Autodesk Inventor part; units mm, degrees
ref_plane "Work Plane2" through (32.2, 0, -89.46) normal (-1, 0, 0) x (0, 0, 1)
ref_plane "YZ Plane" through (0, 0, 0) normal (1, 0, 0) x (0, 1, 0)
ref_plane "XZ Plane" through (0, 0, 0) normal (0, 1, 0) x (-1, 0, 0)
sketch "Sketch1" plane through (0, 0, 0) normal (0, 1, 0) x (-1, 0, 0)
  line L0 (0, 0) -> (-11.7, 0)
  line L1 (-11.7, 0) -> (-11.7, -89.46)
  line L2 (-11.7, -89.46) -> (0, -89.46)
  line L3 (0, -89.46) -> (0, 0)
  line L4 (-26.35, 0) -> (-38.05, 0)
  line L5 (-38.05, 0) -> (-38.05, -89.46)
  line L6 (-38.05, -89.46) -> (-26.35, -89.46)
  line L7 (-26.35, -89.46) -> (-26.35, 0)
  line L8 (-52.7, 0) -> (-64.4, 0)
  line L9 (-64.4, 0) -> (-64.4, -89.46)
  line L10 (-64.4, -89.46) -> (-52.7, -89.46)
  line L11 (-52.7, -89.46) -> (-52.7, 0)
  dimension "d0" = 11.7
  dimension "d1" = 11.7
  dimension "d2" = 11.7
  dimension "d3" = 14.65
  dimension "d4" = 14.65
  dimension "d5" = 89.46
  dimension "d47" = 64.4
extrude "Extrusion1" add sketch "Sketch1" along normal blind 9
sketch "Sketch2" plane through (0, 9, 0) normal (0, 1, 0) x (1, 0, 0)
  line L0 (38.05, 89.46) -> (26.35, 89.46) construction
  line L1 (32.2, 89.46) -> (32.2, 0) construction
  line L2 (26.35, 0) -> (38.05, 0) construction
  line L3 (11.7, 89.46) -> (0, 89.46) construction
  line L4 (5.85, 89.46) -> (5.85, 0) construction
  line L5 (0, 0) -> (11.7, 0) construction
  circle A0 centre (5.85, 84.96) radius 1.5
  circle A1 centre (58.55, 84.96) radius 1.5
  dimension "d8" = 3
  dimension "d9" = 4.5
extrude "Extrusion2" cut sketch "Sketch2" against normal blind 8
sketch "Sketch3" plane through (11.7, 0, -89.46) normal (0, 0, -1) x (-1, 0, 0)
  line L0 (-14.65, 9) -> (-26.35, 9) construction
  line L1 (-20.5, 9) -> (-20.5, 0) construction
  line L2 (-14.65, 0) -> (-26.35, 0) construction
  line L3 (0, 0) -> (11.7, 0)
  line L4 (9.6, 0) -> (9.6, 6.9)
  line L5 (9.6, 6.9) -> (2.1, 6.9)
  line L6 (2.1, 6.9) -> (2.1, 0)
  line L7 (2.1, 0) -> (9.6, 0) construction
  line L8 (0, 0) -> (0, 9) construction
  line L9 (11.7, 0) -> (11.7, 9) construction
  line L10 (-41, 0) -> (-52.7, 0)
  line L11 (-50.6, 0) -> (-50.6, 6.9)
  line L12 (-50.6, 6.9) -> (-43.1, 6.9)
  line L13 (-43.1, 6.9) -> (-43.1, 0)
  dimension "d15" = 7.5
  dimension "d16" = 2.1
  dimension "d17" = 2.1
  dimension "d18" = 6.9
extrude "Extrusion3" cut sketch "Sketch3" against normal through all
sketch "Sketch4" plane through (0, 9, 0) normal (0, 1, 0) x (1, 0, 0)
  line L0 (0, 89.46) -> (0, 0) construction
  line L1 (0, 44.73) -> (64.4, 44.73) construction
  line L2 (64.4, 0) -> (64.4, 89.46) construction
  line L3 (-10, 16) -> (74.4, 16)
  line L4 (74.4, 16) -> (74.4, 19)
  line L5 (74.4, 19) -> (-10, 19)
  line L6 (-10, 19) -> (-10, 16)
  line L7 (-10, 73.46) -> (74.4, 73.46)
  line L8 (74.4, 73.46) -> (74.4, 70.46)
  line L9 (74.4, 70.46) -> (-10, 70.46)
  line L10 (-10, 70.46) -> (-10, 73.46)
  line L11 (52.7, 0) -> (64.4, 0)
  dimension "d21" = 3
  dimension "d22" = 10
  dimension "d23" = 10
  dimension "d46" = 16
extrude "Extrusion4" add sketch "Sketch4" along normal blind 3
ref_plane "Work Plane2" through (32.2, 0, -89.46) normal (-1, 0, 0) x (0, 0, 1)
sketch "Sketch5" plane through (0, 8.5, 0) normal (0, -1, 0) x (1, 0, 0)
  line L0 (23, -75) -> (14, -75)
  line L1 (14, -75) -> (14, -22)
  line L2 (14, -22) -> (23, -22)
  line L3 (23, -22) -> (23, -75)
  line L4 (26, -90) -> (26, 0)
  line L5 (11, 0) -> (11, -90)
  line L6 (11, -22) -> (26, -22)
  line L7 (11, -68) -> (26, -68)
  point P0 (0, 0)
  point P1 (18.5, -22)
  dimension "d27" = 3
  dimension "d28" = 3
  dimension "d29" = 9
  dimension "d30" = 7
sketch "Sketch6" plane through (23, 8.5, -75) normal (0, 0, -1) x (-1, 0, 0)
  line L0 (9, 0) -> (9, -2)
  line L1 (0, 0) -> (0, -2)
  line L2 (9, -0.5) -> (0, -0.5)
  line L3 (0, -0.5) -> (0, -1.5)
  line L4 (0, -1.5) -> (9, -1.5)
  line L5 (9, -1.5) -> (9, -0.5)
  line L6 (9, 0) -> (0, 0)
  line L7 (9, -2) -> (0, -2)
  point P0 (23, -8.5)
  dimension "d34" = 0.5
  dimension "d35" = 0.5
  dimension "d36" = 1
sketch "Sketch7" plane through (14, 8, -75) normal (0, 1, 0) x (1, 0, 0)
  line L0 (1.5, 2) -> (7.5, 2)
  line L1 (7.5, 2) -> (7.5, 4.5)
  line L2 (7.5, 4.5) -> (1.5, 4.5)
  line L3 (1.5, 4.5) -> (1.5, 2)
  line L4 (0, 0) -> (0, 7)
  line L5 (9, 0) -> (9, 7)
  line L6 (0, 7) -> (9, 7)
  point P0 (-14, -75)
  dimension "d39" = 6
  dimension "d40" = 2.5
  dimension "d41" = 1.5
  dimension "d42" = 1.5
  dimension "d43" = 2.5
equation "\"d1\" = d0"
equation "\"d2\" = d1"
equation "\"d4\" = d3"
equation "\"d17\" = d16"
equation "\"d23\" = d22"
equation "\"d28\" = d27"
equation "\"d35\" = d34"
equation "\"d42\" = d41"
properties part number "tracks"
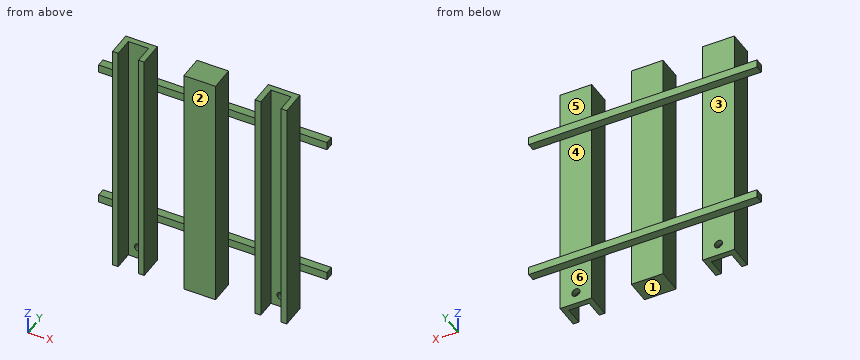
Verification items for the finished model (mm, model axes). Face numbers are marked on the shaded views. A direction names the side the tool comes from. Coordinates: 2 decimals unless noted, no trailing zeros. Loops run counter-clockwise (first coordinate to the right, second up) from the corner with the lowest first, then second, coordinate; pieces in that order, holes last. Notation, with made-up numbers: (79, -19) -> (131, -19) arc R33 cw to (131, 17) -> close; hole circle Ø11 at (62, 41.25). An arc over 180 degrees is marked (long way). Answer in a Markdown table with one row per item.
1) Draft check along Z on the marked faces 1, 2 and 3. Enter one of: released by +Z, released by -Z, zero draft, split by the parting line, or undercut.
The answers:
| item | result |
|---|---|
| face 1 | released by -Z |
| face 2 | zero draft |
| face 3 | undercut |
2) Depth check by flat-ended pin: P1, Ø9.5, axis at x = 60.5, z = -34, coming from the +Y side; P2, Ø2, axis at y = 2, z = -60, coming from the +X side; P3, Ø2.5, axis at x = -3, z = -17.5, coming from the -Y side. Enter the tip coordinate at first touch or a pass-through.
The answers:
| item | result |
|---|---|
| P1 | stops at y = 9 |
| P2 | stops at x = 64.4 |
| P3 | stops at y = 9 |
3) Scan lines: line 1 along X through (y, z) = (5, -38.5); line 2 along X through (y, z) = (7.5, -10); line 3 along Z through (x, y) = (5.85, 7.55). Record each from-to range of solid material in increasing order. Write a range as from..to.
The answers:
| item | result |
|---|---|
| line 1 | x = 0..2.1, 9.6..11.7, 26.35..38.05, 52.7..54.8, 62.3..64.4 |
| line 2 | x = 0..11.7, 26.35..38.05, 52.7..64.4 |
| line 3 | z = -89.46..-86.46, -83.46..0 |
4) Section check B-B (y = 3.25). Record the cut outline in (x, z), and give its area (3 significant figures).
The answers:
| item | result |
|---|---|
| outline | (0, -89.46) -> (2.1, -89.46) -> (2.1, 0) -> (0, 0) -> close; (9.6, -89.46) -> (11.7, -89.46) -> (11.7, 0) -> (9.6, 0) -> close; (26.35, -89.46) -> (38.05, -89.46) -> (38.05, 0) -> (26.35, 0) -> close; (52.7, -89.46) -> (54.8, -89.46) -> (54.8, 0) -> (52.7, 0) -> close; (62.3, -89.46) -> (64.4, -89.46) -> (64.4, 0) -> (62.3, 0) -> close |
| area | 1,800 mm2 |
5) Section check A-A (x = 5.85). Record the cut outline in (y, z).
The answers:
| item | result |
|---|---|
| outline | (6.9, -89.46) -> (9, -89.46) -> (9, -86.46) -> (6.9, -86.46) -> close; (6.9, -83.46) -> (9, -83.46) -> (9, -73.46) -> (12, -73.46) -> (12, -70.46) -> (9, -70.46) -> (9, -19) -> (12, -19) -> (12, -16) -> (9, -16) -> (9, 0) -> (6.9, 0) -> close |
6) Section check C-C (z = -84.96). Record the cut outline in (x, y), and give its area (3 significant figures).
The answers:
| item | result |
|---|---|
| outline | (0, 0) -> (2.1, 0) -> (2.1, 6.9) -> (4.35, 6.9) -> (4.35, 9) -> (0, 9) -> close; (7.35, 6.9) -> (9.6, 6.9) -> (9.6, 0) -> (11.7, 0) -> (11.7, 9) -> (7.35, 9) -> close; (26.35, 0) -> (38.05, 0) -> (38.05, 9) -> (26.35, 9) -> close; (52.7, 0) -> (54.8, 0) -> (54.8, 6.9) -> (57.05, 6.9) -> (57.05, 9) -> (52.7, 9) -> close; (60.05, 6.9) -> (62.3, 6.9) -> (62.3, 0) -> (64.4, 0) -> (64.4, 9) -> (60.05, 9) -> close |
| area | 200 mm2 |
7) Access from +Z, -Z, +X, -X, +Y, -Y to the whole of each face (thin tool, end or side, straight path). Record for the marked faces 4, 5 and 6.
The answers:
| item | result |
|---|---|
| face 4 | +X, -X, +Y |
| face 5 | +Z, +X, -X, +Y |
| face 6 | -Z, +X, -X, +Y |
8) Section check D-D (y = 11). Record the cut outline in (x, z), and give its area (3 significant figures).
The answers:
| item | result |
|---|---|
| outline | (-10, -73.46) -> (74.4, -73.46) -> (74.4, -70.46) -> (-10, -70.46) -> close; (-10, -19) -> (74.4, -19) -> (74.4, -16) -> (-10, -16) -> close |
| area | 506 mm2 |
